Autodesk Inventor part; units mm, degrees
ref_plane "YZ Plane" through (0, 0, 0) normal (1, 0, 0) x (0, 1, 0)
ref_plane "XZ Plane" through (0, 0, 0) normal (0, 1, 0) x (-1, 0, 0)
ref_plane "XY Plane" through (0, 0, 0) normal (0, 0, 1) x (1, 0, 0)
sketch "Sketch1" plane through (0, 0, 0) normal (0, 0, 1) x (1, 0, 0)
  line L0 (0, 0) -> (0, 228.6)
  line L1 (711.2, 0) -> (711.2, 228.6)
  line L2 (266.7, -300.8863) -> (444.5, -300.8863)
  line L3 (355.6, 0) -> (355.6, 228.6)
  line L4 (266.7, 511.9137) -> (444.5, 511.9137)
  line L5 (266.7, 511.9137) -> (0, 228.6)
  line L6 (444.5, 511.9137) -> (711.2, 228.6)
  line L7 (711.2, 0) -> (444.5, -300.8863)
  line L8 (0, 0) -> (266.7, -300.8863)
  point P0 (355.6, -300.8863)
  point P1 (355.6, 511.9137)
  dimension "d39" = 228.6
  dimension "d40" = 711.2
  dimension "d41" = 177.8
  dimension "d42" = 355.6
  dimension "d43" = 177.8
  dimension "d46" = 812.8
  dimension "d47" = 300.8863
extrude "Extrusion1" add sketch "Sketch1" along normal blind 25.4
sketch "Sketch3" plane through (0, 0, 25.4) normal (0, 0, 1) x (1, 0, 0)
  line L0 (444.5, -300.8863) -> (711.2, 0)
  line L1 (711.2, 0) -> (711.2, 228.6)
  line L2 (711.2, 228.6) -> (444.5, 511.9137)
  line L3 (444.5, 511.9137) -> (266.7, 511.9137)
  line L4 (266.7, 511.9137) -> (0, 228.6)
  line L5 (0, 228.6) -> (0, 0)
  line L6 (0, 0) -> (266.7, -300.8863)
  line L7 (266.7, -300.8863) -> (444.5, -300.8863)
  circle A0 centre (419.6269, 499.2137) radius 2.5019
  line L8 (254.7447, 499.2137) -> (456.4553, 499.2137) construction
  circle A1 centre (406.9269, 499.2137) radius 2.5019
  line L9 (242.0447, 499.2137) -> (443.7553, 499.2137) construction
  circle A2 centre (394.2269, 499.2137) radius 2.5019
  line L10 (229.3447, 499.2137) -> (431.0553, 499.2137) construction
  circle A3 centre (381.5269, 499.2137) radius 2.5019
  line L11 (216.6447, 499.2137) -> (418.3553, 499.2137) construction
  circle A4 centre (368.8269, 499.2137) radius 2.5019
  line L12 (203.9447, 499.2137) -> (405.6553, 499.2137) construction
  circle A5 centre (356.1269, 499.2137) radius 2.5019
  line L13 (191.2447, 499.2137) -> (392.9553, 499.2137) construction
  circle A6 centre (343.4269, 499.2137) radius 2.5019
  line L14 (178.5447, 499.2137) -> (380.2553, 499.2137) construction
  circle A7 centre (330.7269, 499.2137) radius 2.5019
  line L15 (165.8447, 499.2137) -> (367.5553, 499.2137) construction
  circle A8 centre (318.0269, 499.2137) radius 2.5019
  line L16 (153.1447, 499.2137) -> (354.8553, 499.2137) construction
  circle A9 centre (305.3269, 499.2137) radius 2.5019
  line L17 (140.4447, 499.2137) -> (342.1553, 499.2137) construction
  circle A10 centre (305.3269, -288.1863) radius 2.5019
  line L18 (305.3269, 499.2137) -> (305.3269, -288.1863) construction
  line L19 (257.0535, -288.1863) -> (455.757, -288.1863) construction
  circle A11 centre (318.0269, -288.1863) radius 2.5019
  line L20 (269.7535, -288.1863) -> (468.457, -288.1863) construction
  circle A12 centre (330.7269, -288.1863) radius 2.5019
  line L21 (282.4535, -288.1863) -> (481.157, -288.1863) construction
  circle A13 centre (343.4269, -288.1863) radius 2.5019
  line L22 (295.1535, -288.1863) -> (493.857, -288.1863) construction
  circle A14 centre (356.1269, -288.1863) radius 2.5019
  line L23 (307.8535, -288.1863) -> (506.557, -288.1863) construction
  circle A15 centre (368.8269, -288.1863) radius 2.5019
  line L24 (320.5535, -288.1863) -> (519.257, -288.1863) construction
  circle A16 centre (381.5269, -288.1863) radius 2.5019
  line L25 (333.2535, -288.1863) -> (531.957, -288.1863) construction
  circle A17 centre (394.2269, -288.1863) radius 2.5019
  line L26 (345.9535, -288.1863) -> (544.657, -288.1863) construction
  circle A18 centre (406.9269, -288.1863) radius 2.5019
  line L27 (358.6535, -288.1863) -> (557.357, -288.1863) construction
  circle A19 centre (419.6269, -288.1863) radius 2.5019
  line L28 (371.3535, -288.1863) -> (570.057, -288.1863) construction
  circle A20 centre (12.7, 206.4884) radius 2.5019
  line L29 (12.7, 242.0911) -> (12.7, -14.3279) construction
  circle A21 centre (12.7, 193.7884) radius 2.5019
  line L30 (12.7, 229.3911) -> (12.7, -27.0279) construction
  circle A22 centre (12.7, 181.0884) radius 2.5019
  line L31 (12.7, 216.6911) -> (12.7, -39.7279) construction
  circle A23 centre (12.7, 168.3884) radius 2.5019
  line L32 (12.7, 203.9911) -> (12.7, -52.4279) construction
  circle A24 centre (12.7, 155.6884) radius 2.5019
  line L33 (12.7, 191.2911) -> (12.7, -65.1279) construction
  circle A25 centre (12.7, 142.9884) radius 2.5019
  line L34 (12.7, 178.5911) -> (12.7, -77.8279) construction
  circle A26 centre (12.7, 130.2884) radius 2.5019
  line L35 (12.7, 165.8911) -> (12.7, -90.5279) construction
  circle A27 centre (12.7, 117.5884) radius 2.5019
  line L36 (12.7, 153.1911) -> (12.7, -103.2279) construction
  circle A28 centre (12.7, 104.8884) radius 2.5019
  line L37 (12.7, 140.4911) -> (12.7, -115.9279) construction
  circle A29 centre (12.7, 92.1884) radius 2.5019
  line L38 (12.7, 127.7911) -> (12.7, -128.6279) construction
  circle A30 centre (12.7, 79.4884) radius 2.5019
  line L39 (12.7, 115.0911) -> (12.7, -141.3279) construction
  circle A31 centre (12.7, 66.7884) radius 2.5019
  line L40 (12.7, 102.3911) -> (12.7, -154.0279) construction
  circle A32 centre (12.7, 54.0884) radius 2.5019
  line L41 (12.7, 89.6911) -> (12.7, -166.7279) construction
  circle A33 centre (12.7, 41.3884) radius 2.5019
  line L42 (12.7, 76.9911) -> (12.7, -179.4279) construction
  circle A34 centre (12.7, 28.6884) radius 2.5019
  line L43 (12.7, 64.2911) -> (12.7, -192.1279) construction
  circle A35 centre (12.7, 15.9884) radius 2.5019
  line L44 (12.7, 51.5911) -> (12.7, -204.8279) construction
  circle A36 centre (12.7, 3.2884) radius 2.5019
  line L45 (12.7, 38.8911) -> (12.7, -217.5279) construction
  circle A37 centre (12.7, -9.4116) radius 2.5019 construction
  line L46 (12.7, 26.1911) -> (12.7, -230.2279) construction
  circle A38 centre (698.5, 206.4884) radius 2.5019
  line L47 (12.7, 206.4884) -> (698.5, 206.4884) construction
  line L48 (698.5, 242.0911) -> (698.5, -14.3279) construction
  circle A39 centre (698.5, 193.7884) radius 2.5019
  circle A40 centre (698.5, 181.0884) radius 2.5019
  circle A41 centre (698.5, 168.3884) radius 2.5019
  circle A42 centre (698.5, 155.6884) radius 2.5019
  circle A43 centre (698.5, 142.9884) radius 2.5019
  circle A44 centre (698.5, 130.2884) radius 2.5019
  circle A45 centre (698.5, 117.5884) radius 2.5019
  circle A46 centre (698.5, 104.8884) radius 2.5019
  circle A47 centre (698.5, 92.1884) radius 2.5019
  circle A48 centre (698.5, 79.4884) radius 2.5019
  circle A49 centre (698.5, 66.7884) radius 2.5019
  circle A50 centre (698.5, 54.0884) radius 2.5019
  circle A51 centre (698.5, 41.3884) radius 2.5019
  circle A52 centre (698.5, 28.6884) radius 2.5019
  circle A53 centre (698.5, 15.9884) radius 2.5019
  circle A54 centre (698.5, 3.2884) radius 2.5019
  circle A55 centre (698.5, -9.4116) radius 2.5019 construction
  dimension "d48" = 5.0038
  dimension "d50" = 12.7
  dimension "d55" = 12.7
  dimension "d60" = 5.0038
  dimension "d61" = 12.7
  dimension "d64" = 12.7
  dimension "d69" = 5.0038
  dimension "d70" = 12.7
  dimension "d73" = 12.7
  dimension "d78" = 5.0038
  dimension "d79" = 12.7
  dimension "d82" = 12.7
extrude "Extrusion2" cut sketch "Sketch3" against normal through all contours A0 | A1 | A2 | A3 | A4 | A5 | A6 | A7 | A8 | A9 | A10 | A11 | A12 | A13 | A14 | A15 | A16 | A17 | A18 | A19 | A20 | A21 | A22 | A23 | A24 | A25 | A26 | A27 | A28 | A29 | A30 | A31 | A32 | A33 | A34 | A35 | A36 | A38 | A39 | A40 | A41 | A42 | A43 | A44 | A45 | A46 | A47 | A48 | A49 | A50 | A51 | A52 | A53 | A54
properties part number "DVBS_008_bellypan" material "Aluminum 6061"
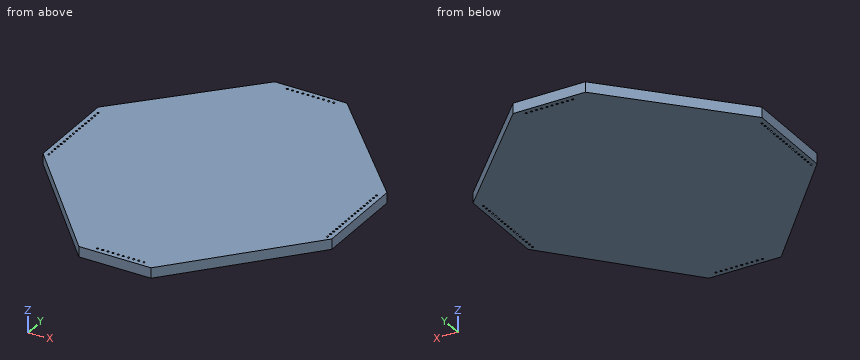
Read the model definition and answer for the solid it produces. Units are mm, in the model's axes. Round coordinates to 2 decimals unless told otherwise and drop trailing zeros. Order: outer loops, then holes, each group sorted by start corner. A loop starts at its lowest first (then second) coordinate and runs counter-clockwise, first axis right, second up.
1) The part is cut by section A-A on y = 370.5. Write down the section's boundary in (x, z).
2) The part is cut by section C-C on z = 11.5. Give the number of separate pieces and of enclosed holes in the cut face, plus the area to 3 significant figures.
3) Straight lines are drawn through the part: L1, parallel to X at y = 119.5, z = 22; L2, parallel to Y at x = 67.5, z = 13.75; L3, parallel to X at y = 425.5, z = 18.5. For each, find the intervals that lie inside material, in ascending order.
4) The part is cut by section B-B on x = 604. Write down the section's boundary in (y, z).
5) Flat-ended cylindrical pins translate along their axes: pin 1 (6 mm diameter, centred on x = 233.5, z = 13.5, fed in from +Y); pin 2 (3 mm diameter, centred on y = -84, z = 4, fed in from +X); pin 3 (1.5 mm diameter, centred on x = 456, z = 7, fed in from -Y). Find the tip coordinate at first contact, or state that the pin passes through.
Resolved:
1. outline: (133.58, 0) - (577.62, 0) - (577.62, 25.4) - (133.58, 25.4) - close
2. separate pieces: 1
2. enclosed holes: 54
2. area: 421,000 mm2
3. L1: x = 0 to 11.09, 14.31 to 696.89, 700.11 to 711.2
3. L2: y = -76.15 to 300.3
3. L3: x = 185.35 to 525.85
4. outline: (-120.94, 0) - (342.48, 0) - (342.48, 25.4) - (-120.94, 25.4) - close
5. pin 1: stops at y = 479.83
5. pin 2: stops at x = 638.07
5. pin 3: stops at y = -288.76
